For this review, take the finished solid that the model builds, in its own axes (mm). Round coordinates to 2 decimals unless told otherwise and drop trailing zeros. Write each loop counter-clockwise with the first axis right and the second up, starting at its lowest first coordinate (ties: lowest second). Pieces come first, ordered by that corner, then holes. Notation, with made-up numbers: M 32,45.25 L 49,45.25 A21 ccw 49,58.25 Z; hole C -1,11.25 d3. An arc over 180 degrees is marked long. One line per question, with ' | ' between items.
```python
from build123d import *

# Parameters (mm, degrees)
SKETCH1_W           = 200
SKETCH1_H           = 127
SKETCH1_R           = 3.96875
SKETCH1_R_2         = 1.6
BOSS_EXTRUDE1_DEPTH = 9.525


with BuildPart() as part:
    # Sketch1 → Boss-Extrude1 (new body)
    with BuildSketch(Plane.XY):
        with Locations((100, 63.5)):
            Rectangle(SKETCH1_W, SKETCH1_H)
        with Locations(Location((66.666666667, 98.425, 0), (0, 0, 180))):
            Circle(SKETCH1_R, mode=Mode.SUBTRACT)
        with Locations(Location((100, 98.425, 0), (0, 0, 180))):
            Circle(SKETCH1_R, mode=Mode.SUBTRACT)
        with Locations(Location((133.333333333, 98.425, 0), (0, 0, 180))):
            Circle(SKETCH1_R, mode=Mode.SUBTRACT)
        with Locations(Location((6, 105, 0), (0, 0, 180))):
            Circle(SKETCH1_R_2, mode=Mode.SUBTRACT)
        with Locations(Location((6, 22, 0), (0, 0, 180))):
            Circle(SKETCH1_R_2, mode=Mode.SUBTRACT)
        with Locations(Location((194, 22, 0), (0, 0, 180))):
            Circle(SKETCH1_R_2, mode=Mode.SUBTRACT)
        with Locations(Location((194, 105, 0), (0, 0, 180))):
            Circle(SKETCH1_R_2, mode=Mode.SUBTRACT)
    extrude(amount=BOSS_EXTRUDE1_DEPTH)


solid = part.part
```
Item 1: To check wall thickness, follow line 1 along X through (y, z) = (105, 3.25); line 2 along Y through (x, z) = (194, 4.25); line 3 along Y through (x, z) = (100, 3). State the ranges of each line that lie inside material, in increasing order. Write a range as from..to.
Results:
line 1: 0..4.4, 7.6..192.4, 195.6..200 | line 2: 0..20.4, 23.6..103.4, 106.6..127 | line 3: 0..94.46, 102.39..127
Item 2: Take a section at B-B (x = 65.5). Write out the cut boundary in (y, z) (3 decimals), then the cut area to 3 significant figures.
Results:
outline: M 0,0 L 94.632,0 L 94.632,9.525 L 0,9.525 Z; M 102.218,0 L 127,0 L 127,9.525 L 102.218,9.525 Z | area: 1,140 mm2
Item 3: Take a section at A-A (x = 100). Write out the cut boundary in (y, z) (3 decimals).
Results:
outline: M 0,0 L 94.456,0 L 94.456,9.525 L 0,9.525 Z; M 102.394,0 L 127,0 L 127,9.525 L 102.394,9.525 Z
Item 4: Mouldability with a two-part tool opening along X and no side actions: class faces 1 (the face through (0, 63, 5)), 2 (the face through (99, 0, 5)), 3 (the face through (129.67, 99.95, 4.7)) as +X half, -X half, draft (parallel to the pull), parting line (faces both ways), or undercut.
Results:
face 1: -X half | face 2: draft | face 3: undercut
